Here's the drawing with two shaded views (mm, measured from the low corner). I have some questions. Round coordinates to 2 decimals unless told otherwise and drop trailing zeros. Loops run counter-clockwise (first coordinate to the right, second up) from the corner with the lowest first, then second, coordinate; pieces in that order, holes last. Notation, with made-up numbers: M -18,62.5 L -14,62.5 A29 ccw -14,95.5 Z; hole C -28,16.5 d4. An arc over 180 degrees is marked long. Answer as CSV lines item,"result".
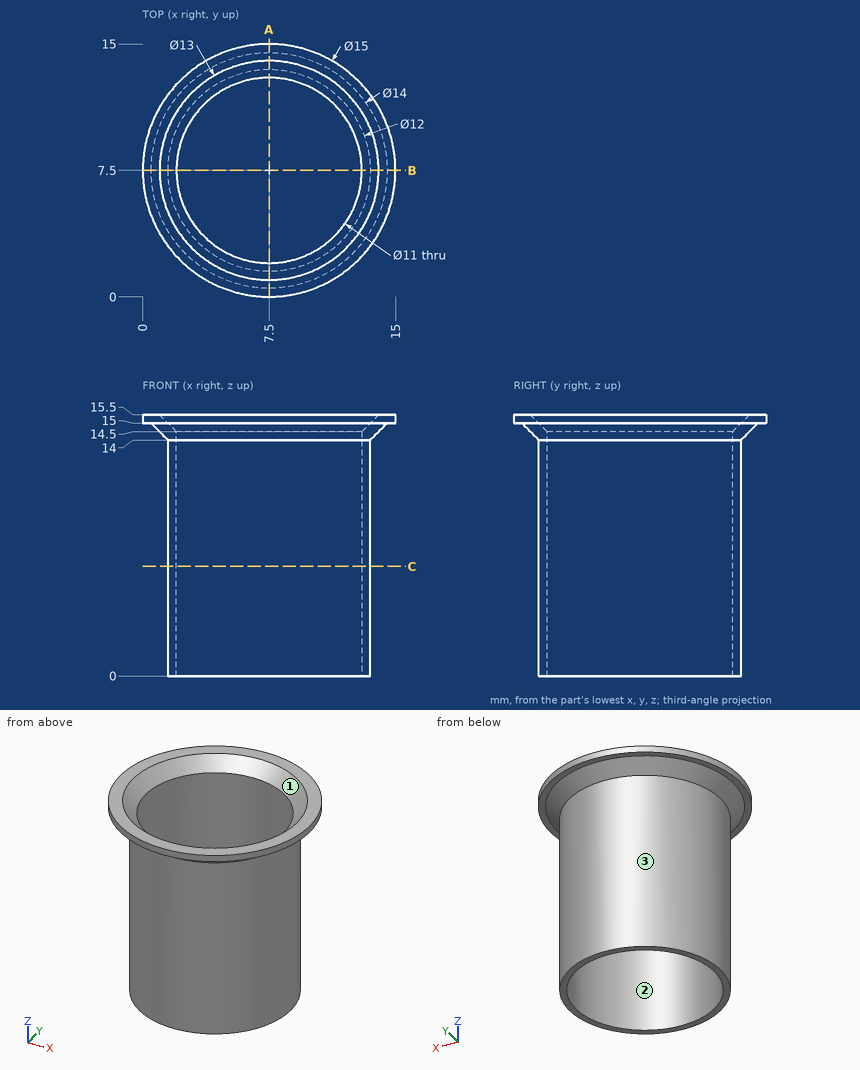
1. I want a section at A-A, the plane x = 7.5. Please give me the cut outline in (y, z), and give its area (3 significant figures).
Evaluation:
outline,"M 0,15 L 0.5,15 L 1.5,14 L 1.5,0 L 2,0 L 2,14.5 L 1,15.5 L 0,15.5 Z; M 13,0 L 13.5,0 L 13.5,14 L 14.5,15 L 15,15 L 15,15.5 L 14,15.5 L 13,14.5 Z"
area,"17.0 mm²"
2. I want a section at C-C, the plane z = 6.5. Please give me the cut outline in (x, y), and give its area (3 significant figures).
Evaluation:
outline,"C 7.5,7.5 d12; hole C 7.5,7.5 d11"
area,"18.1 mm²"
3. If I drill on line 1 (Y direction, x = 7.5, z = 7); line 2 (X direction, y = 8, z = 11); line 3 (Z direction, x = 5.5, y = 14.5), over which ranges is the centre line in solid material (lowest first)? Write a range as [from, to].
Evaluation:
line 1,"y = [1.5, 2], [13, 13.5]"
line 2,"x = [1.52, 2.02], [12.98, 13.48]"
line 3,"z = [15, 15.5]"
4. We'd pull the mould along X, two halves only. Please class the marked faces 1, 2 and 3: pulls with the +X half, pulls with the -X half, needs draft (parallel to the pull), parting line crosses it, or undercut.
Evaluation:
face 1,"undercut"
face 2,"undercut"
face 3,"parting line crosses it"
5. For P1, Ø3, axis at y = 6, z = 7.5, coming from the +X side; P2, Ø3, axis at y = 3, z = 3.5, coming from the -X side; P3, Ø5, axis at x = 5.5, z = 5, coming from the -Y side, each with a flat end and sliding along its axis, tell me the tip position at first contact or that it passes through.
Evaluation:
P1,"stops at x = 13.5"
P2,"stops at x = 2.3"
P3,"stops at y = 1.5"
